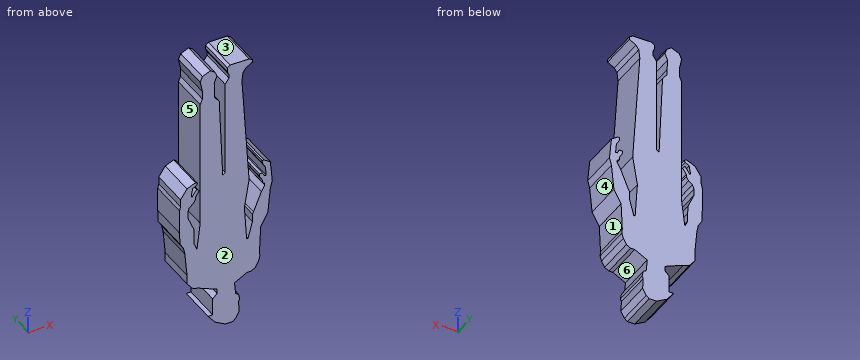
```python
from build123d import *

# Parameters (mm, degrees)
BOSS_EXTRUDE1_DEPTH = 250


with BuildPart() as part:
    # Sketch1 → Boss-Extrude1 (new body)
    with BuildSketch(Plane(origin=(0, 0, 0), x_dir=(1, 0, 0), z_dir=(0, 1, 0))):
        Polygon((578.701410648, 1825.287545316), (531.134778167, 1825.287545316), (465.950874397, 1789.465760361), (421.907696174, 1734.264976989), (451.269814989, 1734.264976989), (451.269814989, 1624.450652619), (478.576585488, 1597.143882121), (478.576585488, 1567.488142118), (359.072761909, 1518.159782508), (323.250976955, 1508.763904487), (287.147809461, 1463.514601229), (287.147809461, 1405.715106095), (273.107994721, 1253.858431719), (265.025038466, 1213.430529779), (242.367567897, 1174.724017557), (239.063353439, 1097.310993114), (239.063353439, 944.824114781), (245.891381344, 918.792258395), (245.891381344, 871.122618446), (287.147809461, 810.289637344), (341.161869432, 786.892336921), (355.466219294, 796.593429505), (348.314044363, 807.139376943), (323.250976955, 821.810440791), (314.154839447, 871.122618446), (318.702908201, 878.892235901), (348.314044363, 835.23034444), (359.072761909, 842.52681831), (364.624616217, 852.011236086), (341.161869432, 886.607271102), (341.161869432, 904.30284394), (326.560938876, 925.832049766), (302.757550724, 944.824114781), (292.128472658, 970.574321762), (292.128472658, 1013.676908453), (330.421956406, 1102.079693826), (332.551821838, 1151.979398219), (332.551821838, 1205.807797227), (350.275497983, 1246.723958017), (371.616569608, 1076.785889831), (371.616569608, 895.455057521), (371.616569608, 260.080879685), (385.440948916, 226.589675052), (385.440948916, 175.377140283), (371.616569608, 106.232803304), (385.847432355, 71.756844149), (436.588755582, 49.777196922), (464.923200239, 68.993384557), (478.576585488, 100.513036666), (460.98809069, 143.123259181), (463.814884827, 209.35100752), (463.814884827, 243.335277368), (493.037068607, 279.960414373), (515.088477789, 796.593429505), (531.134778167, 783.790530267), (531.134778167, 176.23713335), (554.918094408, 141.168415737), (554.918094408, 117.677057814), (545.298983692, 95.470768472), (545.298983692, 68.993384557), (562.942285845, 54.916281775), (684.351522986, 54.916281775), (705.108339961, 68.993384557), (705.108339961, 84.753210612), (662.256489638, 109.837220557), (645.00906552, 135.268705377), (637.979365683, 191.245913613), (683.682414799, 886.607271102), (653.632777579, 1066.724980903), (668.086506196, 1286.63513014), (676.572054292, 1288.050802381), (705.072909907, 1181.809528206), (705.072909907, 1129.77568395), (711.847377196, 1117.44837462), (762.510134993, 994.711812576), (782.850389521, 957.699218271), (782.850389521, 944.824114781), (768.84840262, 935.328082274), (768.84840262, 918.792258395), (750.008410059, 886.607271102), (750.008410059, 869.309253594), (768.84840262, 869.309253594), (782.850389521, 893.22931455), (793.214576246, 893.22931455), (787.8523174, 835.23034444), (768.84840262, 802.765323358), (767.094099882, 783.790530267), (778.35036001, 782.749839711), (819.535342519, 810.681156566), (831.937446607, 944.824114781), (819.535342519, 991.054844082), (803.815773154, 1150.671476587), (757.864939322, 1234.286928314), (750.008410059, 1405.715106095), (752.680318314, 1434.614853662), (743.956821075, 1467.133016429), (724.062751494, 1503.333700421), (697.028330439, 1519.15872738), (670.629087918, 1519.15872738), (590.46447955, 1562.891823116), (597.529835452, 1639.311738223), (616.253387999, 1649.601258091), (623.646904415, 1686.580841707), (616.253387999, 1700.034617481), (620.176367687, 1767.839414568), (597.529835452, 1808.892813111), align=None)
    extrude(amount=BOSS_EXTRUDE1_DEPTH)


solid = part.part
```
Work out the finished part from the listing and answer in its coordinate system (mm). Face numbers are marked on the shaded views. A direction names the side the tool comes from. Give positions to 0.01 mm unless a question says otherwise; leave off trailing zeros. Use one line per item in the form item = value.
1. For the marked faces 1 and 2, determine the directions among +Z, -Z, +X, -X, +Y, -Y from which every point of the face is accessible in a straight line to the end or side of a thin tool.
Filled in:
face_1 = +X, +Y, -Y
face_2 = +Z, -Z, +X, -X, -Y
2. Consider L1, parallel to X at y = 23, z = -1006; L2, parallel to Z at x = 567.5, y = 159.5; L3, parallel to X at y = 101, z = -898. Determine where each line is inside the solid, lowest interval first.
Filled in:
L1 = 239.06 to 292.13, 371.62 to 663.76, 757.85 to 818.06
L2 = -1825.29 to -54.92
L3 = 245.89 to 341.16, 371.62 to 681.78, 756.68 to 827.61
3. Each of these flat-tipped pins is pushed along its axis until it touches: pin 1 Ø10 at (x, y) = (317.5, 61) entering from -Z; pin 2 Ø20.5 at (x, y) = (756, 115.5) entering from +Z; pin 3 Ø13 at (x, y) = (683, 121.5) entering from -Z; pin 4 Ø8 at (x, z) = (529, -1018) entering from -Y. Where does it stop, or does it pass through?
Filled in:
pin_1 = -1507.82
pin_2 = -869.31
pin_3 = -1519.16
pin_4 = 0
4. Determine the mould class of the marked faces 3, 4, 5 and 6 for opening direction Z: released by +Z, released by -Z, zero draft, split by the parting line, or undercut.
Filled in:
face_3 = released by +Z
face_4 = released by -Z
face_5 = zero draft
face_6 = undercut
